Design review of the part built by this model. Coordinates are the model's own, in mm. Face numbers are marked on the shaded views. A direction names the side the tool comes from. Coordinates: 2 decimals unless noted, no trailing zeros. Write each loop counter-clockwise with the first axis right and the second up, starting at its lowest first coordinate (ties: lowest second). Pieces come first, ordered by that corner, then holes.
```python
from build123d import *

# Parameters (mm, degrees)
BOSS_EXTRUDE1_DEPTH = 14
FILLET1_R           = 10
FILLET2_R           = 10
CUT_EXTRUDE1_DEPTH  = 5
SKETCH4_R           = 2.05
CUT_EXTRUDE2_DEPTH  = 78.515972824


with BuildPart() as part:
    # Sketch1 → Boss-Extrude1 (new body)
    with BuildSketch(Plane.XY):
        Polygon((0, 0), (0, 8.92), (18.958818102, 14), (27.958818102, 14), (75.708163648, 3), (75.708163648, 0), align=None)
    extrude(amount=BOSS_EXTRUDE1_DEPTH)

    # Fillet1
    fillet1_edges = [part.edges().sort_by_distance(p)[0] for p in [
        (0, 8.92, 7),
    ]]
    fillet(fillet1_edges, radius=FILLET1_R)

    # Fillet2
    fillet2_edges = [part.edges().sort_by_distance(p)[0] for p in [
        (18.958818102, 14, 7),
        (27.958818102, 14, 7),
    ]]
    fillet(fillet2_edges, radius=FILLET2_R)

    # Sketch3 → Cut-Extrude1 (cut)
    with BuildSketch(Plane.XY.offset(14)):
        Polygon((9.204597923, 0.743591352), (11.254191379, 4.293591352), (9.204597923, 7.843591352), (5.105411012, 7.843591352), (3.055817556, 4.293591352), (5.105411012, 0.743591352), align=None)
        Polygon((25.598194748, 4.356888356), (27.647788204, 7.906888356), (25.598194748, 11.456888356), (21.499007837, 11.456888356), (19.449414382, 7.906888356), (21.499007837, 4.356888356), align=None)
        Polygon((52.17923967, 0.743591352), (54.228833126, 4.293591352), (52.17923967, 7.843591352), (48.080052759, 7.843591352), (46.030459303, 4.293591352), (48.080052759, 0.743591352), align=None)
    extrude(amount=-CUT_EXTRUDE1_DEPTH, mode=Mode.SUBTRACT)

    # Sketch4 → Cut-Extrude2 (cut, through all)
    with BuildSketch(Plane.XY.offset(9)):
        with Locations((7.155004468, 4.293591352)):
            Circle(SKETCH4_R)
        with Locations((23.548601293, 7.906888356)):
            Circle(SKETCH4_R)
        with Locations((50.129646215, 4.293591352)):
            Circle(SKETCH4_R)
    extrude(amount=-CUT_EXTRUDE2_DEPTH, mode=Mode.SUBTRACT)


solid = part.part
```
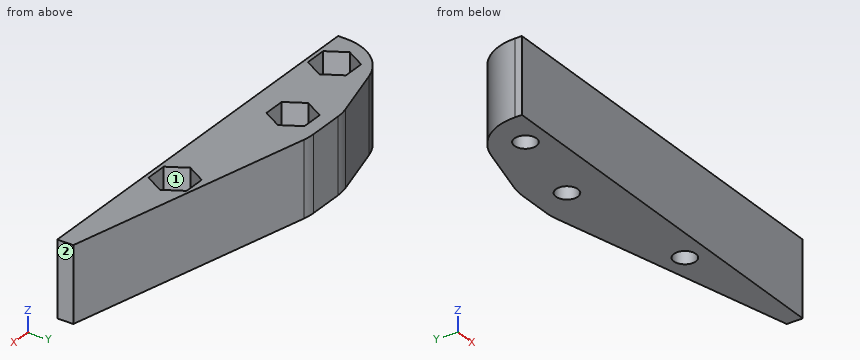
(1) Consider section B-B (z = 12.75). Give the boundary of the cut face in (x, y).
(2) Consider section C-C (x = 60.5). Give the boundary of the cut face in (y, z).
(3) Insertion check: pin 1 Ø3.5 at (x, z) = (7, 11.5) entering from +Y; pin 2 Ø1.2 at (x, z) = (50.5, 12) entering from -Y; pin 3 Ø4.5 at (x, z) = (49, 11.5) entering from +Y. Each pin has a flat end and moves straight along its axis. Give the tip position at first contact, or say it passes through.
(4) Consider section D-D (x = 71). Give the boundary of the cut face in (y, z).
(5) For the marked faces 1 and 2, list the 3-axis set-ups (+Z, -Z, +X, -X, +Y, -Y) from which the entire face can be reached by the end or side of a thin tool; tool diameter is ignored.
(6) Wall thickness on line 1 (Y direction, x = 48.5, z = 4.25); line 2 (Y direction, x = 29.5, z = 11); line 3 (Y direction, x = 66, z = 6.5): over which ranges is each line inside the solid? List them lowest first.
(7) Consider section A-A (z = 2). Give the boundary of the cut face in (x, y) (3 decimals), plus the area to 3 significant figures.
Results:
1. outline: (0, 0) - (75.71, 0) - (75.71, 3) - (29.07, 13.74) arc R10 ccw to (26.82, 14) - (20.28, 14) arc R10 ccw to (17.69, 13.66) - (7.41, 10.91) arc R10 ccw to (0, 1.25) - close; hole (3.06, 4.29) - (5.11, 0.74) - (9.2, 0.74) - (11.25, 4.29) - (9.2, 7.84) - (5.11, 7.84) - close; hole (19.45, 7.91) - (21.5, 4.36) - (25.6, 4.36) - (27.65, 7.91) - (25.6, 11.46) - (21.5, 11.46) - close; hole (46.03, 4.29) - (48.08, 0.74) - (52.18, 0.74) - (54.23, 4.29) - (52.18, 7.84) - (48.08, 7.84) - close
2. outline: (0, 0) - (6.5, 0) - (6.5, 14) - (0, 14) - close
3. pin 1: stops at y = 11.26
3. pin 2: stops at y = 0
3. pin 3: stops at y = 9.67
4. outline: (0, 0) - (4.08, 0) - (4.08, 14) - (0, 14) - close
5. face 1: +Z
5. face 2: +Z, -Z, +X, +Y, -Y
6. line 1: y = 0 to 3.05, 5.54 to 9.27
6. line 2: y = 0 to 13.64
6. line 3: y = 0 to 5.24
7. outline: (0, 0) - (75.708, 0) - (75.708, 3) - (29.067, 13.745) arc R10 ccw to (26.822, 14) - (20.275, 14) arc R10 ccw to (17.687, 13.659) - (7.412, 10.906) arc R10 ccw to (0, 1.247) - close; hole circle Ø4.1 at (7.155, 4.294); hole circle Ø4.1 at (23.549, 7.907); hole circle Ø4.1 at (50.13, 4.294)
7. area: 698 mm2
